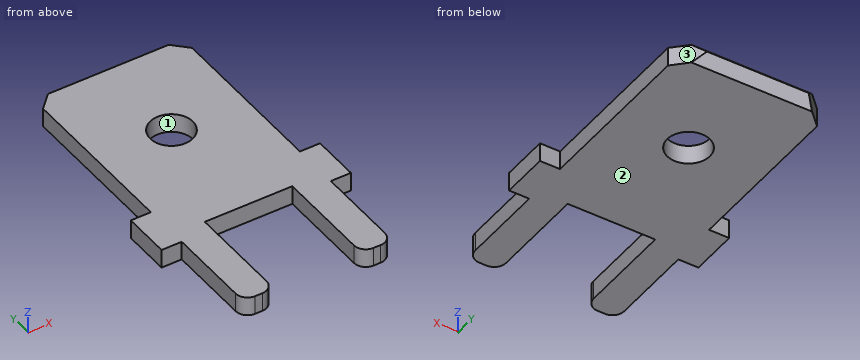
from build123d import *

# Parameters (mm, degrees)
EXTRUSION1_DEPTH   = 0.8
CHANFREIN1_SIZE    = 0.4
CONG_1_R           = 0.5
SKETCH1_R          = 0.9
CUT_EXTRUDE1_DEPTH = 16.45606677


with BuildPart() as part:
    # Esquisse1 → Extrusion1 (new body)
    with BuildSketch(Plane.XY):
        Polygon((-0.65, 0), (0.65, 0), (0.65, 4.5), (4.35, 4.5), (4.35, 0), (5.65, 0), (5.65, 4), (6.5, 4), (6.5, 6), (5.65, 6), (5.65, 13), (4.65, 14), (0.35, 14), (-0.65, 13), (-0.65, 6), (-1.5, 6), (-1.5, 4), (-0.65, 4), align=None)
    extrude(amount=EXTRUSION1_DEPTH)

    # Chanfrein1
    chanfrein1_edges = [part.edges().sort_by_distance(p)[0] for p in [
        (2.5, 14, 0.8),
        (2.5, 14, 0),
    ]]
    chamfer(chanfrein1_edges, length=CHANFREIN1_SIZE - 0.0001)  # a hair under: the kernel refuses the full size

    # Congé1
    cong_1_edges = [part.edges().sort_by_distance(p)[0] for p in [
        (5.65, 0, 0.4),
        (4.35, 0, 0.4),
        (0.65, 0, 0.4),
        (-0.65, 0, 0.4),
    ]]
    fillet(cong_1_edges, radius=CONG_1_R)

    # Sketch1 → Cut-Extrude1 (cut, through all)
    with BuildSketch(Plane.XY.offset(0.8)):
        with Locations((2.5, 9.5)):
            Circle(SKETCH1_R)
    extrude(amount=-CUT_EXTRUDE1_DEPTH, mode=Mode.SUBTRACT)


solid = part.part
Check sheet for the modelled part. Datum: model origin and axes. Units: mm. Face numbers are marked on the shaded views. Give positions to 0.01 mm unless a question says otherwise; leave off trailing zeros. Loops run counter-clockwise (first coordinate to the right, second up) from the corner with the lowest first, then second, coordinate; pieces in that order, holes last. Notation, with made-up numbers: M -27.75,51 L 1.25,51 A10 cw 1.25,62 Z; hole C -11.5,-5.75 d7. An arc over 180 degrees is marked long. Use a Markdown table: item, result. Add a question column.
Q1. Sectioned sample at C-C, the plane z = 0.2. Record the cut outline in (x, y), then the cut area to 3 significant figures.
Q2. Mould release check, pull along X, two halves, no side actions. Record for the marked faces 1, 2 and 3: pulls with the +X half, pulls with the -X half, needs draft (parallel to the pull), parting line crosses it, or undercut.
Q3. Sectioned sample at B-B, the plane y = 9.5. Record the cut outline in (x, z), then the cut area to 3 significant figures.
Q4. Scan lines: line 1 along X through (y, z) = (1.75, 0.55); line 2 along X through (y, z) = (7.25, 0.5). Record each from-to range of solid material in increasing order. Write a range as [from, to].
Verdict:
| question | item | result |
|---|---|---|
| 1 | outline | M -1.5,4 L -0.65,4 L -0.65,0.5 A0.5 ccw -0.15,0 L 0.15,0 A0.5 ccw 0.65,0.5 L 0.65,4.5 L 4.35,4.5 L 4.35,0.5 A0.5 ccw 4.85,0 L 5.15,0 A0.5 ccw 5.65,0.5 L 5.65,4 L 6.5,4 L 6.5,6 L 5.65,6 L 5.65,13 L 4.85,13.8 L 0.15,13.8 L -0.65,13 L -0.65,6 L -1.5,6 Z; hole C 2.5,9.5 d1.8 |
| 1 | area | 70.3 mm^2 |
| 2 | face 1 | undercut |
| 2 | face 2 | needs draft |
| 2 | face 3 | pulls with the +X half |
| 3 | outline | M -0.65,0 L 1.6,0 L 1.6,0.8 L -0.65,0.8 Z; M 3.4,0 L 5.65,0 L 5.65,0.8 L 3.4,0.8 Z |
| 3 | area | 3.60 mm^2 |
| 4 | line 1 | [-0.65, 0.65], [4.35, 5.65] |
| 4 | line 2 | [-0.65, 5.65] |
